The listing builds one solid part. Answer for the finished solid, in the listing's coordinates (mm). A direction names the side the tool comes from. Coordinates: 2 decimals unless noted, no trailing zeros. Loops run counter-clockwise (first coordinate to the right, second up) from the corner with the lowest first, then second, coordinate; pieces in that order, holes last. Notation, with made-up numbers: M 2.5,49 L 31.5,49 A16 ccw 31.5,57 Z; hole C 56.5,59 d4. An arc over 180 degrees is marked long. Return JSON: item names as keys, results as strings. Group by question number.
1. Section C-C (z = -15.75) is taken. Count the separate pieces of the cut face and the enclosed holes in it, then the cut area to 3 significant figures.
2. Section A-A (y = -12) is taken. Write down the section's boundary in (x, z).
3. Section D-D (x = 20) is taken. Write down the section's boundary in (y, z), then the cut area to 3 significant figures.
4. Which of the six approach directions +Z, -Z, +X, -X, +Y, -Y give full straight-line access (tool end or side, diameter ignored) to faces 4 (the face through (2.018, 15.368, -9.014)), 5 (the face through (-16.293, 17.515, -14.056)), 6 (the face through (0, 12, -14))?
5. The mould has two halves that part along X. Classify faces 1 (the face through (29.97, 1.32, -13.94)), 2 (the face through (-20, -6, -10)), 3 (the face through (12, 0, -14)): pulls with the +X half, pulls with the -X half, needs draft (parallel to the pull), parting line crosses it, or undercut.
6. Straight lines are drawn through the part: L1, parallel to Y at x = 0, z = -14.25; L2, parallel to Y at x = 0, z = -13; L3, parallel to Y at x = -1, z = -13. For each, find the intervals that lie inside material, in ascending order. Write a range as from..to.
7. Given P1, Ø8, axis at x = -7, y = -15, coming from the +Z side; P2, Ø0.8, axis at x = 15, z = -17.5, coming from the -Y side; P3, Ø2, axis at x = -4.5, y = -19, coming from the +Z side, each flat-ended and moving along its own axis, determine where each tip first touches the part or whether it passes through.
```python
from build123d import *

# Parameters (mm, degrees)
SKETCH_2_R          = 2.4
EXTRUDE_1_DEPTH     = 3
SKETCH_3_R          = 1.15
EXTRUDE_2_DEPTH     = 3
EXTRUDE_2_2_DEPTH   = 3
EXTRUDE_2_3_DEPTH   = 3
EXTRUDE_2_4_DEPTH   = 3
SKETCH_4_R          = 16
SKETCH_4_R_2        = 15.5
EXTRUDE_3_DEPTH     = 2
SKETCH_5_R          = 30
EXTRUDE_4_DEPTH     = 8
CUT_EXTRUDE_1_REACH = 45.829
SKETCH_6_R          = 4
SKETCH_7_R          = 1
CUT_EXTRUDE_2_DEPTH = 4
SKETCH_9_W          = 1
SKETCH_9_H          = 0.6
CUT_EXTRUDE_3_DEPTH = 1


with BuildPart() as part:
    # Sketch 2 → Extrude 1 (new body)
    with BuildSketch(Plane(origin=(0, 0, -10), x_dir=(-1, 0, 0), z_dir=(0, 0, -1))):
        Circle(SKETCH_2_R)
    extrude(amount=-EXTRUDE_1_DEPTH)



with BuildPart() as body_2:
    # Sketch 3 → Extrude 2 (new body)
    with BuildSketch(Plane(origin=(0, 0, -10), x_dir=(-1, 0, 0), z_dir=(0, 0, -1))):
        with Locations((5.820917719, -1.454962857)):
            Circle(SKETCH_3_R)
    extrude(amount=-EXTRUDE_2_DEPTH)


with BuildPart() as body_3:
    # Sketch 3 → Extrude 2 2 (new body)
    with BuildSketch(Plane(origin=(0, 0, -10), x_dir=(-1, 0, 0), z_dir=(0, 0, -1))):
        with Locations((-1.454962857, -5.820917719)):
            Circle(SKETCH_3_R)
    extrude(amount=-EXTRUDE_2_2_DEPTH)


with BuildPart() as body_4:
    # Sketch 3 → Extrude 2 3 (new body)
    with BuildSketch(Plane(origin=(0, 0, -10), x_dir=(-1, 0, 0), z_dir=(0, 0, -1))):
        with Locations((-5.820917719, 1.454962857)):
            Circle(SKETCH_3_R)
    extrude(amount=-EXTRUDE_2_3_DEPTH)


with BuildPart() as body_5:
    # Sketch 3 → Extrude 2 4 (new body)
    with BuildSketch(Plane(origin=(0, 0, -10), x_dir=(-1, 0, 0), z_dir=(0, 0, -1))):
        with Locations((1.454962857, 5.820917719)):
            Circle(SKETCH_3_R)
    extrude(amount=-EXTRUDE_2_4_DEPTH)


with BuildPart() as body_6:
    # Sketch 4 → Extrude 3 (new body)
    with BuildSketch(Plane(origin=(0, 0, -10), x_dir=(-1, 0, 0), z_dir=(0, 0, -1))):
        Circle(SKETCH_4_R)
        Circle(SKETCH_4_R_2, mode=Mode.SUBTRACT)
    extrude(amount=-EXTRUDE_3_DEPTH)


with BuildPart() as part_1:
    add(part.part)

    add(body_2.part)  # Extrude 4 merges body 2

    add(body_3.part)  # Extrude 4 merges body 3

    add(body_4.part)  # Extrude 4 merges body 4

    add(body_5.part)  # Extrude 4 merges body 5

    add(body_6.part)  # Extrude 4 merges body 6
    # Sketch 5 → Extrude 4 (add)
    with BuildSketch(Plane(origin=(0, 0, -10), x_dir=(-1, 0, 0), z_dir=(0, 0, -1))):
        Circle(SKETCH_5_R)
    extrude(amount=EXTRUDE_4_DEPTH)

    # Sketch 6 → Cut-Extrude 1 (cut, up to next)
    with BuildSketch(Plane(origin=(0, 0, -18), x_dir=(-1, 0, 0), z_dir=(0, 0, -1)), mode=Mode.PRIVATE) as cut_extrude_1_sk1:
        with Locations((0, -20)):
            Circle(SKETCH_6_R)
    cut_extrude_1_tool1 = extrude(cut_extrude_1_sk1.sketch, amount=-CUT_EXTRUDE_1_REACH, mode=Mode.PRIVATE) & part_1.part
    # Sketch 6 → Cut-Extrude 1 (cut, up to next)
    with BuildSketch(Plane(origin=(0, 0, -18), x_dir=(-1, 0, 0), z_dir=(0, 0, -1)), mode=Mode.PRIVATE) as cut_extrude_1_sk2:
        with Locations((-14.142135624, -14.142135624)):
            Circle(SKETCH_6_R)
    cut_extrude_1_tool2 = extrude(cut_extrude_1_sk2.sketch, amount=-CUT_EXTRUDE_1_REACH, mode=Mode.PRIVATE) & part_1.part
    # Sketch 6 → Cut-Extrude 1 (cut, up to next)
    with BuildSketch(Plane(origin=(0, 0, -18), x_dir=(-1, 0, 0), z_dir=(0, 0, -1)), mode=Mode.PRIVATE) as cut_extrude_1_sk3:
        with Locations((-20, 0)):
            Circle(SKETCH_6_R)
    cut_extrude_1_tool3 = extrude(cut_extrude_1_sk3.sketch, amount=-CUT_EXTRUDE_1_REACH, mode=Mode.PRIVATE) & part_1.part
    # Sketch 6 → Cut-Extrude 1 (cut, up to next)
    with BuildSketch(Plane(origin=(0, 0, -18), x_dir=(-1, 0, 0), z_dir=(0, 0, -1)), mode=Mode.PRIVATE) as cut_extrude_1_sk4:
        with Locations((-14.142135624, 14.142135624)):
            Circle(SKETCH_6_R)
    cut_extrude_1_tool4 = extrude(cut_extrude_1_sk4.sketch, amount=-CUT_EXTRUDE_1_REACH, mode=Mode.PRIVATE) & part_1.part
    # Sketch 6 → Cut-Extrude 1 (cut, up to next)
    with BuildSketch(Plane(origin=(0, 0, -18), x_dir=(-1, 0, 0), z_dir=(0, 0, -1)), mode=Mode.PRIVATE) as cut_extrude_1_sk5:
        with Locations((0, 20)):
            Circle(SKETCH_6_R)
    cut_extrude_1_tool5 = extrude(cut_extrude_1_sk5.sketch, amount=-CUT_EXTRUDE_1_REACH, mode=Mode.PRIVATE) & part_1.part
    # Sketch 6 → Cut-Extrude 1 (cut, up to next)
    with BuildSketch(Plane(origin=(0, 0, -18), x_dir=(-1, 0, 0), z_dir=(0, 0, -1)), mode=Mode.PRIVATE) as cut_extrude_1_sk6:
        with Locations((14.142135624, 14.142135624)):
            Circle(SKETCH_6_R)
    cut_extrude_1_tool6 = extrude(cut_extrude_1_sk6.sketch, amount=-CUT_EXTRUDE_1_REACH, mode=Mode.PRIVATE) & part_1.part
    # Sketch 6 → Cut-Extrude 1 (cut, up to next)
    with BuildSketch(Plane(origin=(0, 0, -18), x_dir=(-1, 0, 0), z_dir=(0, 0, -1)), mode=Mode.PRIVATE) as cut_extrude_1_sk7:
        with Locations((20, 0)):
            Circle(SKETCH_6_R)
    cut_extrude_1_tool7 = extrude(cut_extrude_1_sk7.sketch, amount=-CUT_EXTRUDE_1_REACH, mode=Mode.PRIVATE) & part_1.part
    # Sketch 6 → Cut-Extrude 1 (cut, up to next)
    with BuildSketch(Plane(origin=(0, 0, -18), x_dir=(-1, 0, 0), z_dir=(0, 0, -1)), mode=Mode.PRIVATE) as cut_extrude_1_sk8:
        with Locations((14.142135624, -14.142135624)):
            Circle(SKETCH_6_R)
    cut_extrude_1_tool8 = extrude(cut_extrude_1_sk8.sketch, amount=-CUT_EXTRUDE_1_REACH, mode=Mode.PRIVATE) & part_1.part
    add(cut_extrude_1_tool1.solids().sort_by_distance((0, -20, -18))[0], mode=Mode.SUBTRACT)
    add(cut_extrude_1_tool2.solids().sort_by_distance((14.142136, -14.142136, -18))[0], mode=Mode.SUBTRACT)
    add(cut_extrude_1_tool3.solids().sort_by_distance((20, 0, -18))[0], mode=Mode.SUBTRACT)
    add(cut_extrude_1_tool4.solids().sort_by_distance((14.142136, 14.142136, -18))[0], mode=Mode.SUBTRACT)
    add(cut_extrude_1_tool5.solids().sort_by_distance((0, 20, -18))[0], mode=Mode.SUBTRACT)
    add(cut_extrude_1_tool6.solids().sort_by_distance((-14.142136, 14.142136, -18))[0], mode=Mode.SUBTRACT)
    add(cut_extrude_1_tool7.solids().sort_by_distance((-20, 0, -18))[0], mode=Mode.SUBTRACT)
    add(cut_extrude_1_tool8.solids().sort_by_distance((-14.142136, -14.142136, -18))[0], mode=Mode.SUBTRACT)

    # Sketch 7 → Cut-Extrude 2 (cut)
    with BuildSketch(Plane(origin=(0, 0, -18), x_dir=(-1, 0, 0), z_dir=(0, 0, -1))):
        with Locations((12, 0)):
            Circle(SKETCH_7_R)
        with Locations((0, 12)):
            Circle(SKETCH_7_R)
        with Locations((-12, 0)):
            Circle(SKETCH_7_R)
        with Locations((0, -12)):
            Circle(SKETCH_7_R)
    extrude(amount=-CUT_EXTRUDE_2_DEPTH, mode=Mode.SUBTRACT)

    # Sketch 9 → Cut-Extrude 3 (cut)
    with BuildSketch(Plane(origin=(0, 0, -18), x_dir=(-1, 0, 0), z_dir=(0, 0, -1))):
        with Locations((-15, 0)):
            Rectangle(SKETCH_9_W, SKETCH_9_H)
    extrude(amount=-CUT_EXTRUDE_3_DEPTH, mode=Mode.SUBTRACT)


solid = part_1.part
```
Worked out:
{
 "1": {"separate pieces": "1", "enclosed holes": "12", "area": "2,410 mm^2"},
 "2": {"outline": "M -27.5,-18 L -17.52,-18 L -17.52,-10 L -27.5,-10 Z; M -10.76,-18 L -1,-18 L -1,-14 L 1,-14 L 1,-18 L 10.76,-18 L 10.76,-10 L 10.58,-10 L 10.58,-8 L 9.81,-8 L 9.81,-10 L -9.81,-10 L -9.81,-8 L -10.58,-8 L -10.58,-10 L -10.76,-10 Z; M 17.52,-18 L 27.5,-18 L 27.5,-10 L 17.52,-10 Z"},
 "3": {"outline": "M -22.36,-18 L -4,-18 L -4,-10 L -22.36,-10 Z; M 4,-18 L 22.36,-18 L 22.36,-10 L 4,-10 Z", "area": "294 mm^2"},
 "4": {"face 4": "+Z", "face 5": "+Z, -Z", "face 6": "-Z"},
 "5": {"face 1": "parting line crosses it", "face 2": "needs draft", "face 3": "undercut"},
 "6": {"L1": "-30..-24, -16..-13, -11..11, 13..16, 24..30", "L2": "-30..-24, -16..16, 24..30", "L3": "-29.98..-23.87, -16.13..16.13, 23.87..29.98"},
 "7": {"P1": "z = -8", "P2": "y = -26.21", "P3": "z = -10"}
}
